The model under review builds one solid part; all positions refer to its coordinate system, in mm. A direction names the side the tool comes from. Coordinates: 2 decimals unless noted, no trailing zeros. Write each loop counter-clockwise with the first axis right and the second up, starting at its lowest first coordinate (ties: lowest second). Pieces come first, ordered by that corner, then holes. Notation, with made-up numbers: M 39,-31 L 97,-31 A21 cw 97,-7 Z; hole C 54.5,21 d6. An arc over 180 degrees is marked long. Answer as CSV lines item,"result". Start each with the question number.
from build123d import *

# Parameters (mm, degrees)
SKETCH3_W           = 25.7
SKETCH3_H           = 39.2
SKETCH3_W_2         = 14.4
SKETCH3_H_2         = 29.9
BOSS_EXTRUDE2_DEPTH = 12
CHAMFER1_SIZE       = 1
CHAMFER1_SIZE2      = 10


with BuildPart() as part:
    # Sketch3 → Boss-Extrude2 (new body)
    with BuildSketch(Plane.XY):
        with Locations((12.85, 19.6)):
            Rectangle(SKETCH3_W, SKETCH3_H)
        with Locations((12.85, 19.6)):
            Rectangle(SKETCH3_W_2, SKETCH3_H_2, mode=Mode.SUBTRACT)
    extrude(amount=BOSS_EXTRUDE2_DEPTH)

    # Chamfer1
    chamfer1_edges = [part.edges().sort_by_distance(p)[0] for p in [
        (5.65, 19.6, 0),
        (12.85, 4.65, 0),
        (20.05, 19.6, 0),
        (12.85, 34.55, 0),
        (12.85, 39.2, 0),
        (25.7, 19.6, 0),
        (12.85, 0, 0),
        (0, 19.6, 0),
    ]]
    chamfer1_side = [part.faces().sort_by_distance(p)[0] for p in [
        (12.85, 0.468735533, 0),
    ]]
    chamfer(chamfer1_edges, length=CHAMFER1_SIZE, length2=CHAMFER1_SIZE2, reference=chamfer1_side[0])

    # Sweep1: sweep along a path in Sketch6
    with BuildLine(Plane.ZY.offset(-12.85)) as sweep1_path:
        Line((12, 4.65), (24.033327649, -2.297444957))
    # Sketch4 → Sweep1 (sweep)
    with BuildSketch(Plane.XY.offset(12)):
        Polygon((5.65, 10.65), (2.65, 10.65), (2.65, 1.65), (23.05, 1.65), (23.05, 10.65), (20.05, 10.65), (20.05, 4.65), (5.65, 4.65), align=None)
    sweep(path=sweep1_path.line)


solid = part.part
1) Clearance check with flat-ended pins moving along their axes: pin 1 Ø3.5 at (y, z) = (3.5, 20.5) entering from +X; pin 2 Ø1.6 at (x, z) = (15, 11) entering from -Y; pin 3 Ø13 at (x, y) = (18, 18.5) entering from +Z; pin 4 Ø8 at (y, z) = (23, 15) entering from -X. State where each tip first meets the part, or that it passes through.
2) To check wall thickness, follow line 1 (X direction, y = 32, z = 11); line 2 (X direction, y = 4.5, z = 14.25); line 3 (Z direction, x = 24.5, y = 14). State the ranges of each line that lie inside material, in increasing order. Write a range as [from, to].
3) Take a section at A-A on y = 22.5. Give the boundary of the cut face in (x, z), and give its area (3 significant figures).
4) Take a section at D-D on z = 2.5. Give the boundary of the cut face in (x, y), and give its area (3 significant figures).
5) Mouldability with a two-part tool opening along Y and no side actions: class faces 1 (the flat face through (12.95, 1.13, 18.1)), 2 (the flat face through (0.493, 19.326, 5.07)), 3 (the flat face through (20.05, 9, 14)) as +Y half, -Y half, draft (parallel to the pull), parting line (faces both ways), or undercut.
6) Take a section at B-B on z = 8. Give the boundary of the cut face in (x, y), and give its area (3 significant figures).
7) Take a section at C-C on x = 19.5. Give the boundary of the cut face in (y, z).
8) Tool access review of faces 4 (the flat face through (5.157, 19.377, 5.07)), 5 (the flat face through (13, 34.55, 11)), 6 (the flat face through (5.65, 9, 14)), 7 (the flat face through (23.05, 3, 18)): name each direction out of +Z, -Z, +X, -X, +Y, -Y from which nothing blocks a thin tool from reaching the whole face with its end or side.
Results:
1,pin 1,"stops at x = 23.05"
1,pin 2,"stops at y = 0"
1,pin 3,"stops at z = 12"
1,pin 4,"stops at x = 0"
2,line 1,"x = [0, 5.65], [20.05, 25.7]"
2,line 2,"x = [2.65, 5.65], [20.05, 23.05]"
2,line 3,"z = [0, 12]"
3,outline,"M 0,10 L 1,0 L 4.65,0 L 5.65,10 L 5.65,12 L 0,12 Z; M 20.05,10 L 21.05,0 L 24.7,0 L 25.7,10 L 25.7,12 L 20.05,12 Z"
3,area,"116 mm²"
4,outline,"M 0.75,0.75 L 24.95,0.75 L 24.95,38.45 L 0.75,38.45 Z; hole M 4.9,3.9 L 20.8,3.9 L 20.8,35.3 L 4.9,35.3 Z"
4,area,"413 mm²"
5,face 1,"+Y half"
5,face 2,"draft"
5,face 3,"undercut"
6,outline,"M 0.2,0.2 L 25.5,0.2 L 25.5,39 L 0.2,39 Z; hole M 5.45,4.45 L 20.25,4.45 L 20.25,34.75 L 5.45,34.75 Z"
6,area,"533 mm²"
7,outline,"M -5.3,24.03 L 1.65,12 L 0,12 L 0,10 L 1,0 L 3.65,0 L 4.65,10 L 4.65,12 L -2.3,24.03 Z; M 34.55,10 L 35.55,0 L 38.2,0 L 39.2,10 L 39.2,12 L 34.55,12 Z"
8,face 4,"-Z"
8,face 5,"+Z, -Z"
8,face 6,"+Z"
8,face 7,"+Z, +X, +Y, -Y"
